```python
from build123d import *

# Parameters (mm, degrees)
SKETCH1_R           = 1.5
BOSS_EXTRUDE1_DEPTH = 1
SKETCH3_W           = 22.58
SKETCH3_H           = 12
SKETCH3_W_2         = 6
SKETCH3_H_2         = 4
BOSS_EXTRUDE2_DEPTH = 2.8
SKETCH4_W           = 8.26
SKETCH4_H           = 4.16
BOSS_EXTRUDE3_DEPTH = 4.25


with BuildPart() as part:
    # Sketch1 → Boss-Extrude1 (new body)
    with BuildSketch(Plane.XY):
        with BuildLine():
            Line((-73.608329156, 15.618710575), (-51.028329156, 15.618710575))
            ThreePointArc((-51.028329156, 15.618710575), (-44.528329156, 22.118710575), (-51.028329156, 28.618710575))
            Line((-51.028329156, 28.618710575), (-73.608329156, 28.618710575))
            ThreePointArc((-73.608329156, 28.618710575), (-80.108329156, 22.118710575), (-73.608329156, 15.618710575))
        make_face()
        with Locations((-76.818329156, 22.118710575)):
            Circle(SKETCH1_R, mode=Mode.SUBTRACT)
        with Locations(Location((-47.818329156, 22.118710575, 0), (0, 0, 180))):
            Circle(SKETCH1_R, mode=Mode.SUBTRACT)
    extrude(amount=BOSS_EXTRUDE1_DEPTH)

    # Sketch3 → Boss-Extrude2 (add)
    with BuildSketch(Plane(origin=(0, 0, 0), x_dir=(-1, 0, 0), z_dir=(0, 0, -1))):
        with Locations((62.318329156, 22.118710575)):
            Rectangle(SKETCH3_W, SKETCH3_H)
        with Locations((58.090026235, 22.118710575)):
            Rectangle(SKETCH3_W_2, SKETCH3_H_2, mode=Mode.SUBTRACT)
    extrude(amount=BOSS_EXTRUDE2_DEPTH)

    # Sketch4 → Boss-Extrude3 (add)
    with BuildSketch(Plane.XY.offset(1)):
        with Locations((-68.460165602, 26.538710575)):
            Rectangle(SKETCH4_W, SKETCH4_H)
        with Locations((-56.176492709, 26.538710575)):
            Rectangle(SKETCH4_W, SKETCH4_H)
    extrude(amount=BOSS_EXTRUDE3_DEPTH)


solid = part.part
```
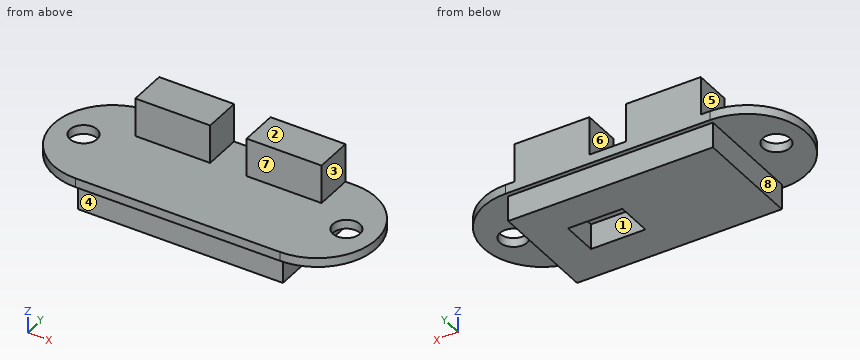
Check sheet for the modelled part. Datum: model origin and axes. Units: mm. Face numbers are marked on the shaded views. A direction names the side the tool comes from. Give positions to 0.01 mm unless a question says otherwise; leave off trailing zeros. Loops run counter-clockwise (first coordinate to the right, second up) from the corner with the lowest first, then second, coordinate; pieces in that order, holes last. Notation, with made-up numbers: (70, -14) - (81, -14) arc R18 ccw to (81, -7) - close; hole circle Ø5 at (-4.75, 11). An arc over 180 degrees is marked (long way). One line per question, with ' | ' between items. Start each with the question number.
1. Draft check along X on the marked faces 1, 2 and 3. Enter one of: released by +X, released by -X, zero draft, split by the parting line, or undercut.
2. Material ranges on line 1 along X through (y, z) = (26.5, 2.75); line 2 along X through (y, z) = (21.5, -1); line 3 along Y through (x, z) = (-57, -2), recorded low to high. Write a range as [from, to].
3. Cross-section at A-A, the plane z = 2.5. Enter the section's corners in (x, y), plus the area to 3 significant figures.
4. Gauge pin test, flat ends, axial feed: pin 1 Ø0.8 at (x, z) = (-67.5, -2) entering from -Y; pin 2 Ø3.5 at (x, z) = (-57, 4) entering from -Y; pin 3 Ø1 at (y, z) = (25, 3.5) entering from -X; pin 4 Ø1 at (x, z) = (-74.5, 4) entering from -Y. Record the tip position at first contact, or that the pin passes through.
5. Set-up check for the marked faces 4, 5, 6, 7 and 8: record each of +Z, -Z, +X, -X, +Y, -Y from which the full face is reachable in a straight line by a thin tool's end or side.
6. Cross-section at B-B, the plane y = 23. Enter the section's corners in (x, z), plus the area to 3 significant figures.
7. Cross-section at C-C, the plane z = -2. Enter the section's corners in (x, y).
8. Cross-section at D-D, the plane x = -63.5. Enter the section's corners in (y, z).
Check result:
1) face 1: undercut | face 2: zero draft | face 3: released by +X
2) line 1: x = [-72.59, -64.33], [-60.31, -52.05] | line 2: x = [-73.61, -61.09], [-55.09, -51.03] | line 3: y = [16.12, 20.12], [24.12, 28.12]
3) outline: (-72.59, 24.46) - (-64.33, 24.46) - (-64.33, 28.62) - (-72.59, 28.62) - close; (-60.31, 24.46) - (-52.05, 24.46) - (-52.05, 28.62) - (-60.31, 28.62) - close | area: 68.7 mm2
4) pin 1: stops at y = 16.12 | pin 2: stops at y = 24.46 | pin 3: stops at x = -72.59 | pin 4: passes through
5) face 4: -Z, +X, -X, -Y | face 5: +Z, -X, +Y, -Y | face 6: +Z, +Y, -Y | face 7: +Z, +X, -X, -Y | face 8: -Z, -X, +Y, -Y
6) outline: (-80.05, 0) - (-78.03, 0) - (-78.03, 1) - (-80.05, 1) - close; (-75.6, 0) - (-73.61, 0) - (-73.61, -2.8) - (-61.09, -2.8) - (-61.09, 0) - (-55.09, 0) - (-55.09, -2.8) - (-51.03, -2.8) - (-51.03, 0) - (-49.03, 0) - (-49.03, 1) - (-75.6, 1) - close; (-46.6, 0) - (-44.59, 0) - (-44.59, 1) - (-46.6, 1) - close | area: 77.0 mm2
7) outline: (-73.61, 16.12) - (-51.03, 16.12) - (-51.03, 28.12) - (-73.61, 28.12) - close; hole (-61.09, 20.12) - (-55.09, 20.12) - (-55.09, 24.12) - (-61.09, 24.12) - close
8) outline: (15.62, 0) - (16.12, 0) - (16.12, -2.8) - (28.12, -2.8) - (28.12, 0) - (28.62, 0) - (28.62, 1) - (15.62, 1) - close
